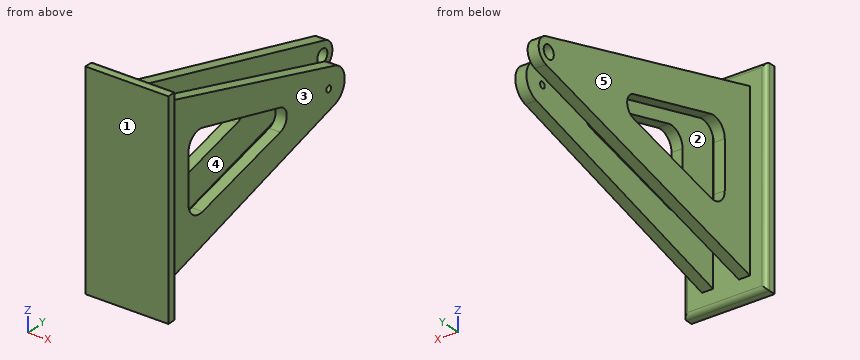
Autodesk Inventor part; units mm, degrees
ref_plane "Work Plane1" through (51.2805, 0, 22.9336) normal (1, 0, 0) x (0, 0, -1)
ref_plane "Work Plane2" through (5.0525, 0, -176.9644) normal (-1, 0, 0) x (0, 0, 1)
ref_plane "YZ Plane" through (0, 0, 0) normal (1, 0, 0) x (0, 1, 0)
sketch "Sketch1" plane through (0, 0, 0) normal (0, 1, 0) x (-1, 0, 0)
  line L0 (10.6955, 22.9336) -> (-69.3145, 22.9336)
  line L1 (-69.3145, 22.9336) -> (-69.3145, -176.9644)
  line L2 (-69.3145, -176.9644) -> (10.6955, -176.9644)
  line L3 (10.6955, -176.9644) -> (10.6955, 22.9336)
  point P0 (0, 0)
  dimension "d0" = 80.01
  dimension "d1" = 199.898
extrude "Extrusion1" add sketch "Sketch1" along normal blind 10.668
fillet "Fillet1" radius 4.064 4 edges at (29.3095, 10.668, 22.9336) (69.3145, 10.668, -77.0154) (29.3095, 10.668, -176.9644) (-10.6955, 10.668, -77.0154)
ref_plane "Work Plane1" through (51.2805, 0, 22.9336) normal (1, 0, 0) x (0, 0, -1)
sketch "Sketch2" plane through (51.2805, 0, 22.9336) normal (1, 0, 0) x (0, 0, -1)
  line L0 (195.834, 10.668) -> (4.064, 10.668) construction
  line L1 (195.834, 10.668) -> (183.134, 10.668) construction
  arc A0 (4.064, 10.668) -> (0, 6.604) centre (4.064, 6.604) ccw construction
  line L2 (4.064, 10.668) -> (16.764, 10.668) construction
  line L3 (82.8788, 237.5782) -> (16.764, 10.668)
  line L4 (183.134, 10.668) -> (117.0192, 237.5782)
  line L5 (77.1008, 49.7952) -> (122.7972, 49.7952)
  line L6 (136.8055, 67.9313) -> (110.7624, 167.66)
  line L7 (89.1356, 167.66) -> (63.0925, 67.9313)
  arc A1 (117.0192, 237.5782) -> (82.8788, 237.5782) centre (99.949, 232.6044) ccw
  arc A2 (110.7624, 167.66) -> (89.1356, 167.66) centre (99.949, 164.8362) ccw
  arc A3 (63.0925, 67.9313) -> (77.1008, 49.7952) centre (77.1008, 64.2732) ccw
  arc A4 (122.7972, 49.7952) -> (136.8055, 67.9313) centre (122.7972, 64.2732) ccw
  line L8 (16.764, 10.668) -> (183.134, 10.668)
  point P0 (22.9336, 0)
  dimension "d6" = 12.7
  dimension "d7" = 12.7
  dimension "d9" = 17.78
  dimension "d10" = 11.176
  dimension "d11" = 14.478
extrude "Extrusion2" add sketch "Sketch2" against normal blind 10.668
sketch "Sketch3" plane through (51.2805, 0, 22.9336) normal (1, 0, 0) x (0, 0, -1)
  line L0 (16.764, 10.668) -> (183.134, 10.668)
  circle A0 centre (99.949, 229.8407) radius 3.048
  point P0 (22.9336, 0)
  dimension "d15" = 6.096
extrude "Extrusion3" cut sketch "Sketch3" against normal up to next
ref_plane "Work Plane2" through (5.0525, 0, -176.9644) normal (-1, 0, 0) x (0, 0, 1)
sketch "Sketch4" plane through (5.0525, 0, -176.9644) normal (-1, 0, 0) x (0, 0, 1)
  line L0 (16.764, 10.668) -> (183.134, 10.668)
  line L1 (117.0192, 237.5782) -> (183.134, 10.668)
  line L2 (16.764, 10.668) -> (183.134, 10.668)
  line L3 (16.764, 10.668) -> (87.4428, 272.4493)
  line L4 (112.4552, 272.4493) -> (183.134, 10.668)
  line L5 (16.764, 10.668) -> (183.134, 10.668)
  line L6 (77.1396, 43.0817) -> (122.7584, 43.0817)
  line L7 (136.7593, 61.2458) -> (110.7567, 160.0105)
  line L8 (89.1413, 160.0105) -> (63.1387, 61.2458)
  arc A0 (110.7567, 160.0105) -> (89.1413, 160.0105) centre (99.949, 157.1651) ccw
  arc A1 (63.1387, 61.2458) -> (77.1396, 43.0817) centre (77.1396, 57.5597) ccw
  arc A2 (122.7584, 43.0817) -> (136.7593, 61.2458) centre (122.7584, 57.5597) ccw
  line L9 (16.764, 10.668) -> (183.134, 10.668)
  arc A3 (112.4552, 272.4493) -> (87.4428, 272.4493) centre (99.949, 269.0728) ccw
  point P0 (176.9644, 0)
  point P1 (99.949, 318.77)
  point P2 (99.949, 201.0611)
  dimension "d21" = 11.176
  dimension "d22" = 14.478
  dimension "d25" = 12.954
extrude "Extrusion4" add sketch "Sketch4" against normal blind 10.668
sketch "Sketch5" plane through (5.0525, 0, -176.9644) normal (-1, 0, 0) x (0, 0, 1)
  arc A0 (112.4552, 272.4493) -> (87.4428, 272.4493) centre (99.949, 269.0728) ccw
  circle A1 centre (99.949, 269.0728) radius 6.477
  point P0 (176.9644, 0)
  dimension "d26" = 12.954
extrude "Extrusion5" cut sketch "Sketch5" against normal up to next
properties part number "Stand"
The listing builds one solid part. Answer for the finished solid, in the listing's coordinates (mm). Face numbers are marked on the shaded views. A direction names the side the tool comes from. Coordinates: 2 decimals unless noted, no trailing zeros. Order: outer loops, then holes, each group sorted by start corner. A loop starts at its lowest first (then second) coordinate and runs counter-clockwise, first axis right, second up. Notation, with made-up numbers: M -26.5,-29 L 25.5,-29 A22 ccw 25.5,-20 Z; hole C 87.5,12.25 d2. An arc over 180 degrees is marked long. Use CSV: the item, a comma, the result in double quotes.
Q1. Section D-D (x = 31.5) is taken. Determine the outline of the cut face in (y, z), then the cut area to 3 significant figures.
Here are the results:
outline,"M 0,-176.96 L 6.6,-176.96 A4.06 ccw 10.67,-172.9 L 10.67,18.87 A4.06 ccw 6.6,22.93 L 0,22.93 Z"
area,"2,130 mm2"
Q2. Section B-B (z = -44) is taken. Determine the outline of the cut face in (x, y), then the cut area to 3 significant figures.
Here are the results:
outline,"M -10.7,0 L 69.31,0 L 69.31,6.6 A4.06 ccw 65.25,10.67 L 51.28,10.67 L 51.28,53.97 L 40.61,53.97 L 40.61,10.67 L 15.72,10.67 L 15.72,47.29 L 5.05,47.29 L 5.05,10.67 L -6.63,10.67 A4.06 ccw -10.7,6.6 Z; M 5.05,75.66 L 15.72,75.66 L 15.72,196.49 L 5.05,196.49 Z; M 40.61,82.64 L 51.28,82.64 L 51.28,182.85 L 40.61,182.85 Z"
area,"4,060 mm2"
Q3. Straight lines are drawn through the part: L1, parallel to Y at x = 31, z = -93; L2, parallel to X at y = 244, z = -59; L3, parallel to X at y = 21.5, z = -84. For each, find the intervals that lie inside material, in ascending order.
Here are the results:
L1,"0 to 10.67"
L2,"5.05 to 15.72"
L3,"5.05 to 15.72, 40.61 to 51.28"
Q4. A tool of negligible diameter and unlimited length cuts with its end or side. For the marked faces 1 and 2, from which of +Z, -Z, +X, -X, +Y, -Y can it reach the whole face along a straight path? Write none if from no direction.
Here are the results:
face 1,"+Z, -Z, +X, -X, -Y"
face 2,"+Z, -Z, +Y"
Q5. Section A-A (y = 203) is taken. Determine the outline of the cut face in (x, z), then the cut area to 3 significant figures.
Here are the results:
outline,"M 5.05,-108.27 L 15.72,-108.27 L 15.72,-45.76 L 5.05,-45.76 Z; M 40.61,-104.16 L 51.28,-104.16 L 51.28,-49.87 L 40.61,-49.87 Z"
area,"1,250 mm2"
Q6. Given pin 1 Ø20.5 at (y, z) = (269.07, -77.02) entering from +X; pin 2 Ø2 at (x, z) = (28.5, -148) entering from +Y; pin 3 Ø6 at (y, z) = (74, -39) entering from -X, each flat-ended and moving along its own axis, determine where each tip first touches the part or whether it passes through.
Here are the results:
pin 1,"x = 15.72"
pin 2,"y = 10.67"
pin 3,"x = 5.05"
Q7. Determine the mould class of the marked faces 3, 4 and 5 for opening direction X: pulls with the +X half, pulls with the -X half, needs draft (parallel to the pull), parting line crosses it, or undercut.
Here are the results:
face 3,"pulls with the +X half"
face 4,"undercut"
face 5,"pulls with the -X half"
Q8. Section C-C (y = 125) is taken. Determine the outline of the cut face in (x, z), then the cut area to 3 significant figures.
Here are the results:
outline,"M 5.05,-129.33 L 15.72,-129.33 L 15.72,-97.04 L 5.05,-97.04 Z; M 5.05,-56.99 L 15.72,-56.99 L 15.72,-24.7 L 5.05,-24.7 Z; M 40.61,-126.89 L 51.28,-126.89 L 51.28,-98.97 L 40.61,-98.97 Z; M 40.61,-55.06 L 51.28,-55.06 L 51.28,-27.14 L 40.61,-27.14 Z"
area,"1,280 mm2"
